Can you work these out from the model? Positions are in its coordinate system, mm. Give positions to 0.01 mm unless a question says otherwise; leave off trailing zeros. Loops run counter-clockwise (first coordinate to the right, second up) from the corner with the lowest first, then second, coordinate; pieces in that order, holes last. Notation, with made-up numbers: M 44.25,28 L 57.25,28 A25 ccw 57.25,50 Z; hole C 75,54 d2. An arc over 180 degrees is marked long. Answer as a JSON object with one key per item and string values.
```python
from build123d import *

# Parameters (mm, degrees)
F0_R     = 12.7
F1_DEPTH = 4.7625
F2_SIZE  = 2.38124


# Not quite as in the source:
# - a fillet or chamfer is up to 0.001 mm smaller than in the source, because OpenCascade refuses the exact size


with BuildPart() as f1:
    # F0 (on Top) → F1 (new body)
    with BuildSketch(Plane.XY):
        with BuildLine():
            Line((-19.05, 31.75), (-19.05, 0))
            ThreePointArc((-19.05, 0), (-13.4703841816, -13.4703841816), (0, -19.05))
            Line((0, -19.05), (79.375, -19.05))
            ThreePointArc((79.375, -19.05), (92.8453841816, -13.4703841816), (98.425, 0))
            Line((98.425, 0), (98.425, 31.75))
            ThreePointArc((98.425, 31.75), (69.05625, 22.225), (39.6875, 31.75))
            ThreePointArc((39.6875, 31.75), (10.31875, 22.225), (-19.05, 31.75))
        make_face()
        Circle(F0_R, mode=Mode.SUBTRACT)
        with BuildLine():
            Line((79.375, -12.7), (28.575, -12.7))
            ThreePointArc((28.575, -12.7), (15.875, 0), (28.575, 12.7))
            Line((28.575, 12.7), (79.375, 12.7))
            ThreePointArc((79.375, 12.7), (92.075, 0), (79.375, -12.7))
        make_face(mode=Mode.SUBTRACT)
    extrude(amount=F1_DEPTH)

    # F2 (size 2.38125 in the source; OpenCascade refuses exactly that, so slightly less here)
    f2_edges = [f1.edges().sort_by_distance(p)[0] for p in [
        (10.31875, 22.225, 4.7625),
        (69.05625, 22.225, 4.7625),
        (69.05625, 22.225, 0),
        (10.31875, 22.225, 0),
    ]]
    chamfer(f2_edges, length=F2_SIZE)


solid = f1.part
```
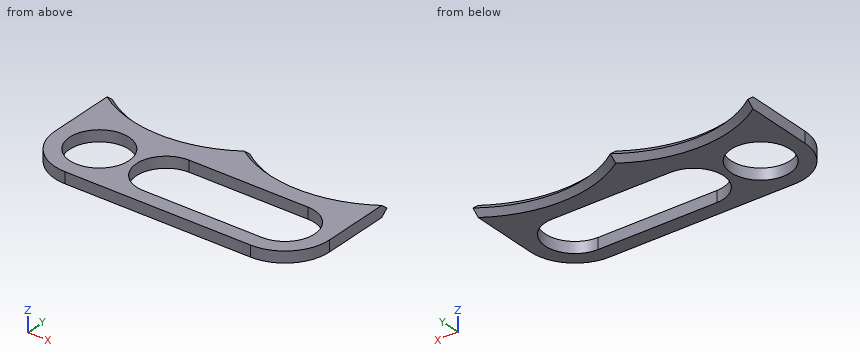
1) Will this pin go through, and if not, where does the flat tip stop? pin 1 Ø2.5 at (x, z) = (42, 1.5) entering from +Y.
Answer list:
{"pin 1": "y = 30.75"}
2) Suppose I cut it at B-B, the plane z = 3.6. Give the number of separate pieces and of enclosed holes in the cut face, and give its area (3 significant figures).
Answer list:
{"separate pieces": "1", "enclosed holes": "2", "area": "2,590 mm^2"}
3) Suppose I cut it at D-D, the plane y = -16. Write out the boundary of the cut face in (x, z).
Answer list:
{"outline": "M -10.34,0 L 89.71,0 L 89.71,4.76 L -10.34,4.76 Z"}
4) Please list where these lines run through material, in increasing order: line 1 along Y through (x, z) = (85.5, 4.15); line 2 along X through (y, z) = (9, 3.4) (3 decimals); line 3 along Y through (x, z) = (34.5, 3.4). Write a range as from..to.
Answer list:
{"line 1": "-18.04..-11.13, 11.13..23.14", "line 2": "-19.05..-8.96, 8.96..19.615, 88.335..98.425", "line 3": "-19.05..-12.7, 12.7..27.3"}
5) Suppose I cut it at A-A, the plane y = -9. Write out the boundary of the cut face in (x, z), and give its area (3 significant figures).
Answer list:
{"outline": "M -16.79,0 L -8.96,0 L -8.96,4.76 L -16.79,4.76 Z; M 8.96,0 L 19.61,0 L 19.61,4.76 L 8.96,4.76 Z; M 88.34,0 L 96.16,0 L 96.16,4.76 L 88.34,4.76 Z", "area": "125 mm^2"}
